Design review of the part built by this model. Coordinates are the model's own, in mm. Coordinates: 2 decimals unless noted, no trailing zeros. Loops run counter-clockwise (first coordinate to the right, second up) from the corner with the lowest first, then second, coordinate; pieces in that order, holes last.
from build123d import *

# Parameters (mm, degrees)
SKETCH1_R           = 32
BOSS_EXTRUDE1_DEPTH = 3
SKETCH2_R           = 10
CUT_EXTRUDE1_DEPTH  = 10
SKETCH3_R           = 1.5
CUT_EXTRUDE2_DEPTH  = 4


with BuildPart() as part:
    # Sketch1 → Boss-Extrude1 (new body)
    with BuildSketch(Plane(origin=(0, 0, 0), x_dir=(1, 0, 0), z_dir=(0, 1, 0))):
        Circle(SKETCH1_R)
    extrude(amount=BOSS_EXTRUDE1_DEPTH)

    # Sketch2 → Cut-Extrude1 (cut)
    with BuildSketch(Plane(origin=(0, 3, 0), x_dir=(1, 0, 0), z_dir=(0, 1, 0))):
        Circle(SKETCH2_R)
    extrude(amount=-CUT_EXTRUDE1_DEPTH, mode=Mode.SUBTRACT)

    # Sketch3 → Cut-Extrude2 (cut, through all)
    with BuildSketch(Plane.XZ):
        with Locations((13, 0)):
            Circle(SKETCH3_R)
        with Locations((0, -13)):
            Circle(SKETCH3_R)
        with Locations((-13, 0)):
            Circle(SKETCH3_R)
        with Locations((0, 13)):
            Circle(SKETCH3_R)
    extrude(amount=-CUT_EXTRUDE2_DEPTH, mode=Mode.SUBTRACT)


solid = part.part
Q1. For line 1 (Z direction, x = 0, y = 2.35); line 2 (Z direction, x = 1, y = 0.4); line 3 (Z direction, x = 13, y = 1), list the stretches that pass through material, from the lowest coordinate up.
Q2. Take a section at A-A, the plane x = 0. Write out the cut boundary in (y, z), then the cut area to 3 significant figures.
Q3. Take a section at B-B, the plane x = 9. Write out the cut boundary in (y, z).
Q4. Take a section at C-C, the plane y = 1.15. Write out the cut boundary in (x, z).
Q5. The part is to be moulded in two halves that separate along Z. For faces 1 (the cylindrical face through (-6.94, 1.48, 31.24)), 2 (the cylindrical face through (-14.5, 1.48, 0.07)), 3 (the flat face through (7, 0, -8)), say which applies: pulls with the +Z half, pulls with the -Z half, needs draft (parallel to the pull), parting line crosses it, or undercut.
Q6. Clearance check with a flat-ended pin moving along its axis: pin 1 Ø16 at (x, z) = (0, 0) entering from -Y. State where the tip first meets the part, or that it passes through.
Q7. Take a section at D-D, the plane z = 13. Write out the cut boundary in (x, y).
Entries:
1. line 1: z = -32 to -14.5, -11.5 to -10, 10 to 11.5, 14.5 to 32
1. line 2: z = -31.98 to -14.12, -11.88 to -9.95, 9.95 to 11.88, 14.12 to 31.98
1. line 3: z = -29.24 to -1.5, 1.5 to 29.24
2. outline: (0, -32) - (3, -32) - (3, -14.5) - (0, -14.5) - close; (0, -11.5) - (3, -11.5) - (3, -10) - (0, -10) - close; (0, 10) - (3, 10) - (3, 11.5) - (0, 11.5) - close; (0, 14.5) - (3, 14.5) - (3, 32) - (0, 32) - close
2. area: 114 mm2
3. outline: (0, -30.71) - (3, -30.71) - (3, -4.36) - (0, -4.36) - close; (0, 4.36) - (3, 4.36) - (3, 30.71) - (0, 30.71) - close
4. outline: circle Ø64 at (0, 0); hole circle Ø3 at (-13, 0); hole circle Ø20 at (0, 0); hole circle Ø3 at (0, -13); hole circle Ø3 at (0, 13); hole circle Ø3 at (13, 0)
5. face 1: parting line crosses it
5. face 2: undercut
5. face 3: needs draft
6. pin 1: passes through
7. outline: (-29.24, 0) - (-1.5, 0) - (-1.5, 3) - (-29.24, 3) - close; (1.5, 0) - (29.24, 0) - (29.24, 3) - (1.5, 3) - close
